```python
from build123d import *

# Parameters (mm, degrees)
SKIZZE1_W                       = 110
SKIZZE1_H                       = 110
AUFSATZ_LINEAR_AUSTRAGEN1_DEPTH = 41
VERRUNDUNG1_R                   = 15
SCHNITT_LINEAR_AUSTRAGEN1_DEPTH = 111
KREISMUSTER1_COUNT              = 2
KREISMUSTER1_ANGLE              = 90


with BuildPart() as part:
    # Skizze1 → Aufsatz-Linear austragen1 (new body)
    with BuildSketch(Plane(origin=(0, 0, 0), x_dir=(1, 0, 0), z_dir=(0, 1, 0))):
        Rectangle(SKIZZE1_W, SKIZZE1_H)
    extrude(amount=-AUFSATZ_LINEAR_AUSTRAGEN1_DEPTH)

    # Verrundung1
    verrundung1_edges = [part.edges().sort_by_distance(p)[0] for p in [
        (55, -20.5, 55),
        (-55, -20.5, 55),
        (-55, -20.5, -55),
        (55, -20.5, -55),
    ]]
    fillet(verrundung1_edges, radius=VERRUNDUNG1_R)

    # Skizze2 → Schnitt-Linear austragen1 (cut, through all)
    with BuildSketch(Plane.XY.offset(55)):
        with BuildLine():
            Line((-30.5, -41), (-30.5, -37))
            ThreePointArc((-30.5, -37), (-29.621320344, -34.878679656), (-27.5, -34))
            Line((-27.5, -34), (27.5, -34))
            ThreePointArc((27.5, -34), (29.621320344, -34.878679656), (30.5, -37))
            Line((30.5, -37), (30.5, -41))
            Line((30.5, -41), (-30.5, -41))
        make_face()
    schnitt_linear_austragen1 = extrude(amount=-SCHNITT_LINEAR_AUSTRAGEN1_DEPTH, mode=Mode.SUBTRACT)

    # Kreismuster1: Schnitt-Linear austragen1 ×2 about axis
    kreismuster1_axis = Axis((0, -43.05, 0), (0, 1, 0))
    for i in range(1, KREISMUSTER1_COUNT):
        add(schnitt_linear_austragen1.rotate(kreismuster1_axis, i * KREISMUSTER1_ANGLE / (KREISMUSTER1_COUNT - 1)), mode=Mode.SUBTRACT)


solid = part.part
```
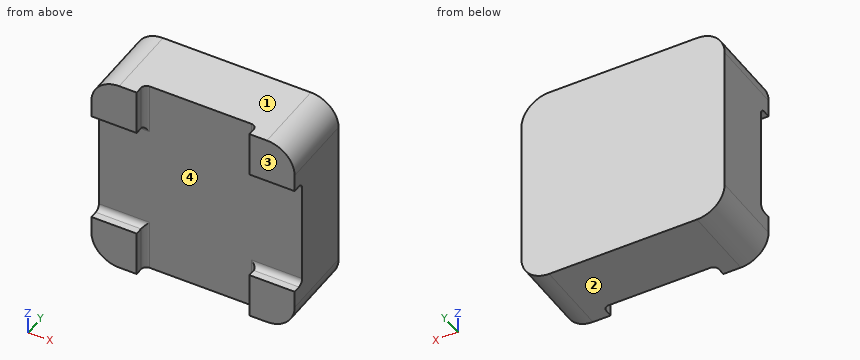
Check sheet for the modelled part. Datum: model origin and axes. Units: mm. Face numbers are marked on the shaded views. Round coordinates to 2 decimals unless told otherwise and drop trailing zeros. Order: outer loops, then holes, each group sorted by start corner. A loop starts at its lowest first (then second) coordinate and runs counter-clockwise, first axis right, second up. Notation, with made-up numbers: (79, -30.5) - (89, -30.5) arc R15 ccw to (89, -7.5) - close; hole circle Ø9 at (27.25, 87). An arc over 180 degrees is marked (long way). Answer as CSV lines item,"result". Start each with the question number.
1) Section check A-A (y = -32). Record the cut outline in (x, z), then the cut area to 3 significant figures.
2) Draft check along Z on the marked faces 1, 2, 3 and 4. Enter one of: +Z half, -Z half, draft (parallel to the pull), parting line (faces both ways), or undercut.
3) Depth check by flat-ended pin: pin 1 (3 mm diameter, centred on y = -39.5, z = 49, fed in from -X); pin 2 (3 mm diameter, centred on x = 42, y = -39.5, fed in from +Z); pin 3 (4 mm diameter, centred on x = 16, z = 42.5, fed in from +Y); pin 4 (1.2 mm diameter, centred on x = -45, y = -39, fed in from -Z). Enter the tip coordinate at first touch or a pass-through.
4) Section check C-C (z = 25.5). Record the cut outline in (x, y).
5) Section check D-D (z = -47.5). Record the cut outline in (x, y).
6) Scan lines: probe 1 along Y at (x, z) = (-1, 27.5); probe 2 along Z at (x, y) = (-33.5, -37); probe 3 along Z at (x, y) = (-30.5, -35.5). Record each from-to range of solid material in increasing order.
7) Section check B-B (x = -34.5). Record the cut outline in (y, z), then the cut area to 3 significant figures.
Determined:
1,outline,"(-55, -40) arc R15 ccw to (-40, -55) - (40, -55) arc R15 ccw to (55, -40) - (55, 40) arc R15 ccw to (40, 55) - (-40, 55) arc R15 ccw to (-55, 40) - close"
1,area,"11,900 mm^2"
2,face 1,"+Z half"
2,face 2,"-Z half"
2,face 3,"draft"
2,face 4,"undercut"
3,pin 1,"x = -52.99"
3,pin 2,"z = 54.99"
3,pin 3,"y = 0"
3,pin 4,"z = -54.34"
4,outline,"(-55, -34) - (55, -34) - (55, 0) - (-55, 0) - close"
5,outline,"(-52.99, -41) - (-30.5, -41) - (-30.5, -37) arc R3 cw to (-27.5, -34) - (27.5, -34) arc R3 cw to (30.5, -37) - (30.5, -41) - (52.99, -41) - (52.99, 0) - (-52.99, 0) - close"
6,probe 1,"-34 to 0"
6,probe 2,"-55 to -30.5, 30.5 to 55"
6,probe 3,"-55 to -30.1, 30.1 to 55"
7,outline,"(-41, -55) - (0, -55) - (0, 55) - (-41, 55) - (-41, 30.5) - (-37, 30.5) arc R3 cw to (-34, 27.5) - (-34, -27.5) arc R3 cw to (-37, -30.5) - (-41, -30.5) - close"
7,area,"4,090 mm^2"
